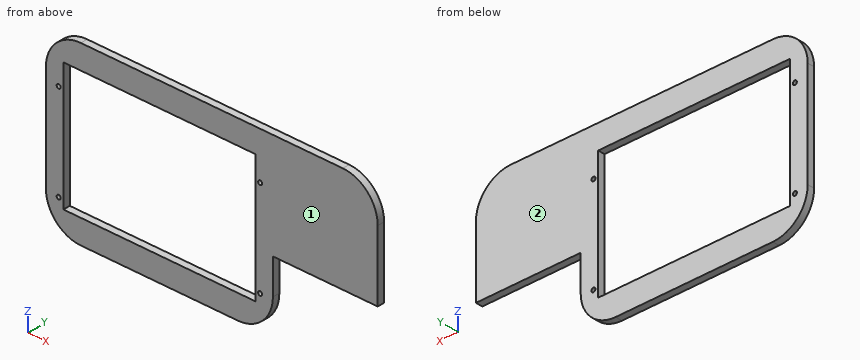
```python
from build123d import *

# Parameters (mm, degrees)
SKETCH1_W           = 165
SKETCH1_H           = 109
BOSS_EXTRUDE1_DEPTH = 6
SKETCH2_R           = 1.75
CUT_EXTRUDE4_DEPTH  = 323.119543027


with BuildPart() as part:
    # Sketch1 → Boss-Extrude1 (new body)
    with BuildSketch(Plane(origin=(0, 0, 0), x_dir=(1, 0, 0), z_dir=(0, 1, 0))):
        with BuildLine():
            Line((30, 150), (165, 150))
            ThreePointArc((165, 150), (186.213203436, 141.213203436), (195, 120))
            Line((195, 120), (195, 90))
            Line((195, 90), (285, 90))
            Line((285, 90), (285, 30))
            ThreePointArc((285, 30), (276.213203436, 8.786796564), (255, 0))
            Line((255, 0), (30, 0))
            ThreePointArc((30, 0), (8.786796564, 8.786796564), (0, 30))
            Line((0, 30), (0, 120))
            ThreePointArc((0, 120), (8.786796564, 141.213203436), (30, 150))
        make_face()
        with Locations((97.5, 75)):
            Rectangle(SKETCH1_W, SKETCH1_H, mode=Mode.SUBTRACT)
    extrude(amount=BOSS_EXTRUDE1_DEPTH)

    # Sketch2 → Cut-Extrude4 (cut, through all)
    with BuildSketch(Plane(origin=(0, 0, 0), x_dir=(1, 0, 0), z_dir=(0, 1, 0))):
        with Locations(Location((184, 122.05, 0), (0, 0, 90))):
            Circle(SKETCH2_R)
        with Locations(Location((11, 122.05, 0), (0, 0, 270))):
            Circle(SKETCH2_R)
        with Locations(Location((184, 39.95, 0), (0, 0, 270))):
            Circle(SKETCH2_R)
        with Locations(Location((11, 39.95, 0), (0, 0, 90))):
            Circle(SKETCH2_R)
    extrude(amount=CUT_EXTRUDE4_DEPTH, mode=Mode.SUBTRACT)


solid = part.part
```
CAD build for the part. Positions are in the model's coordinates, mm. Face numbers are marked on the shaded views. Give positions to 0.01 mm unless a question says otherwise; leave off trailing zeros. Write each loop counter-clockwise with the first axis right and the second up, starting at its lowest first coordinate (ties: lowest second). Pieces come first, ordered by that corner, then holes. Notation, with made-up numbers: M 8.5,-18.5 L 48.5,-18.5 A28 ccw 48.5,10.5 Z; hole C -21,-19.75 d2. An arc over 180 degrees is marked long. Return JSON: item names as keys, results as strings. Group by question number.
(1) Band-saw the part on C-C (y = 2.6). Give the cut face in (x, z), and give its area (3 significant figures).
(2) Band-saw the part on A-A (z = -112). Give the cut face in (x, y), and give its area (3 significant figures).
(3) Band-saw the part on D-D (x = 207). Give the cut face in (y, z).
(4) Mould opens along Y. For the marked faces 1 and 2 say: pulls with the +Y half, pulls with the -Y half, needs draft (parallel to the pull), parting line crosses it, or undercut.
(5) Drill centre lines: L1, parallel to X at y = 1.65, z = -39.95; L2, parallel to X at y = 1.3, z = -50.5; L3, parallel to Z at x = 109.5, y = 3.3. Where is each one in solid material? Low to high. Write a range as [from, to].
(6) Band-saw the part on B-B (x = 149). Give the cut face in (y, z), and give its area (3 significant figures).
(7) Flat gauge pins, fed straight in: pin 1 Ø2 at (x, y) = (212, 3) entering from -Z; pin 2 Ø4 at (x, z) = (184, -39.95) entering from -Y; pin 3 Ø1.8 at (y, z) = (2, -101.5) entering from +X. Where does each tip first touch, or does it go through?
Entries:
{
 "1": {"outline": "M 0,-120 A30 ccw 30,-150 L 165,-150 A30 ccw 195,-120 L 195,-90 L 285,-90 L 285,-30 A30 ccw 255,0 L 30,0 A30 ccw 0,-30 Z; hole C 11,-122.05 d3.5; hole C 11,-39.95 d3.5; hole M 15,-129.5 L 180,-129.5 L 180,-20.5 L 15,-20.5 Z; hole C 184,-122.05 d3.5; hole C 184,-39.95 d3.5", "area": "18,600 mm^2"},
 "2": {"outline": "M 0,0 L 15,0 L 15,6 L 0,6 Z; M 180,0 L 195,0 L 195,6 L 180,6 Z", "area": "180 mm^2"},
 "3": {"outline": "M 0,-90 L 6,-90 L 6,0 L 0,0 Z"},
 "4": {"face 1": "pulls with the -Y half", "face 2": "pulls with the +Y half"},
 "5": {"L1": "x = [0, 9.25], [12.75, 15], [180, 182.25], [185.75, 285]", "L2": "x = [0, 15], [180, 285]", "L3": "z = [-150, -129.5], [-20.5, 0]"},
 "6": {"outline": "M 0,-150 L 6,-150 L 6,-129.5 L 0,-129.5 Z; M 0,-20.5 L 6,-20.5 L 6,0 L 0,0 Z", "area": "246 mm^2"},
 "7": {"pin 1": "stops at z = -90", "pin 2": "stops at y = 0", "pin 3": "stops at x = 195"}
}
